Can you work these out from the model? Positions are in its coordinate system, mm. Round coordinates to 2 decimals unless told otherwise and drop trailing zeros. Loops run counter-clockwise (first coordinate to the right, second up) from the corner with the lowest first, then second, coordinate; pieces in that order, holes last. Notation, with made-up numbers: (31, 22.25) -> (84, 22.25) arc R27 cw to (84, 45.25) -> close; hole circle Ø11 at (-31.5, -0.75). An arc over 180 degrees is marked (long way). Answer as a JSON object with one key per item and string values.
```python
from build123d import *

# Parameters (mm, degrees)
BOSS_EXTRUDE1_DEPTH  = 8
M4_CLEARANCE_HOLE1_D = 4.3
SKETCH4_W            = 80
SKETCH4_H            = 3.5
CUT_EXTRUDE1_DEPTH   = 10
M4_CLEARANCE_HOLE2_D = 4.3


with BuildPart() as part:
    # Sketch1 → Boss-Extrude1 (new body)
    with BuildSketch(Plane(origin=(0, 0, 0), x_dir=(1, 0, 0), z_dir=(0, 1, 0))):
        Polygon((-40, 80.5), (-40, 0), (-40, -80.5), (40, -80.5), (40, 80.5), align=None)
    extrude(amount=BOSS_EXTRUDE1_DEPTH)

    # M4 Clearance Hole1 (through all)
    with Locations(Plane(origin=(0, 8, 0), x_dir=(1, 0, 0), z_dir=(0, 1, 0))):
        with Locations((-26.5, 57), (26.5, 57), (-26.5, 39), (26.5, 39), (26.5, -39), (-26.5, -39), (26.5, -57), (-26.5, -57)):
            Hole(M4_CLEARANCE_HOLE1_D / 2)

    # Sketch4 → Cut-Extrude1 (cut)
    with BuildSketch(Plane(origin=(0, 8, 0), x_dir=(1, 0, 0), z_dir=(0, 1, 0))):
        with Locations((0, 78.75)):
            Rectangle(SKETCH4_W, SKETCH4_H)
        with Locations((0, -78.75)):
            Rectangle(SKETCH4_W, SKETCH4_H)
    extrude(amount=-CUT_EXTRUDE1_DEPTH, mode=Mode.SUBTRACT)

    # M4 Clearance Hole2 (through all)
    with Locations(Plane(origin=(0, 8, 0), x_dir=(1, 0, 0), z_dir=(0, 1, 0))):
        with Locations((-17, 0), (0, 17), (17, 0), (0, -17)):
            Hole(M4_CLEARANCE_HOLE2_D / 2)


solid = part.part
```
Q1. I want a section at B-B, the plane z = -17. Write out the boundary of the cut face in (x, y).
Determined:
{"outline": "(-40, 0) -> (-2.15, 0) -> (-2.15, 8) -> (-40, 8) -> close; (2.15, 0) -> (40, 0) -> (40, 8) -> (2.15, 8) -> close"}
Q2. I want a section at C-C, the plane x = 26.5. Write out the boundary of the cut face in (y, z).
Determined:
{"outline": "(0, -77) -> (8, -77) -> (8, -59.15) -> (0, -59.15) -> close; (0, -54.85) -> (8, -54.85) -> (8, -41.15) -> (0, -41.15) -> close; (0, -36.85) -> (8, -36.85) -> (8, 36.85) -> (0, 36.85) -> close; (0, 41.15) -> (8, 41.15) -> (8, 54.85) -> (0, 54.85) -> close; (0, 59.15) -> (8, 59.15) -> (8, 77) -> (0, 77) -> close"}
Q3. If I drill on L1, parallel to Z at x = 26.5, y = 3.75; L2, parallel to X at y = 3.75, z = 39; L3, parallel to Z at x = 17, y = 3.5, over which ranges is the centre line in solid material (lowest first)? Write a range as [from, to].
Determined:
{"L1": "[-77, -59.15], [-54.85, -41.15], [-36.85, 36.85], [41.15, 54.85], [59.15, 77]", "L2": "[-40, -28.65], [-24.35, 24.35], [28.65, 40]", "L3": "[-77, -2.15], [2.15, 77]"}
Q4. We'd pull the mould along Z, two halves only. Please class faces 1 (the cylindrical face through (26.78, 3.94, -41.13)), 2 (the flat face through (-1, 4, 77)), 3 (the flat face through (-1, 4, -77)), 4 (the flat face through (40, 4, 1)): pulls with the +Z half, pulls with the -Z half, needs draft (parallel to the pull), parting line crosses it, or undercut.
Determined:
{"face 1": "undercut", "face 2": "pulls with the +Z half", "face 3": "pulls with the -Z half", "face 4": "needs draft"}
Q5. I'm going to push flat-ended pins straight in: pin 1 (4 mm diameter, centred on x = -26.5, z = 57, fed in from -Y); pin 2 (2 mm diameter, centred on x = 25, z = 31, fed in from -Y). Where does each tip first touch, or does it pass through?
Determined:
{"pin 1": "through", "pin 2": "y = 0"}
Q6. I want a section at A-A, the plane x = -17. Write out the boundary of the cut face in (y, z).
Determined:
{"outline": "(0, -77) -> (8, -77) -> (8, -2.15) -> (0, -2.15) -> close; (0, 2.15) -> (8, 2.15) -> (8, 77) -> (0, 77) -> close"}
Q7. I want a section at D-D, the plane z = 0. Write out the boundary of the cut face in (x, y).
Determined:
{"outline": "(-40, 0) -> (-19.15, 0) -> (-19.15, 8) -> (-40, 8) -> close; (-14.85, 0) -> (14.85, 0) -> (14.85, 8) -> (-14.85, 8) -> close; (19.15, 0) -> (40, 0) -> (40, 8) -> (19.15, 8) -> close"}
